Work out the finished part from the listing and answer in its coordinate system (mm). A direction names the side the tool comes from. Give positions to 0.01 mm unless a question says otherwise; leave off trailing zeros. Loops run counter-clockwise (first coordinate to the right, second up) from the corner with the lowest first, then second, coordinate; pieces in that order, holes last.
```python
from build123d import *

# Parameters (mm, degrees)
F0_W      = 82.55
F0_H      = 63.5
F1_DEPTH  = 15.748
F3_DEPTH  = 4.064
F4_W      = 19.05
F4_H      = 63.5
F5_DEPTH  = 4.826
F7_DEPTH  = 19.05
F8_R      = 6.35
F9_DEPTH  = 8.89
F14_DEPTH = 25.4
F16_DEPTH = 25.4
F18_W     = 23.9344900474
F18_H     = 17.6518000662
F19_DEPTH = 31.75


with BuildPart() as f1:
    # F0 (on Top) → F1 (new body)
    with BuildSketch(Plane.XY):
        Rectangle(F0_W, F0_H)
    extrude(amount=F1_DEPTH)

    # F2 (on face) → F3 (cut)
    with BuildSketch(Plane.XY.offset(15.748)):
        Polygon((-41.275, 1.4794587481), (-15.875, 31.75), (-41.275, 31.75), align=None)
    extrude(amount=-F3_DEPTH, mode=Mode.SUBTRACT)

    # F4 (on face) → F5 (join)
    with BuildSketch(Plane(origin=(0, 0, 0), x_dir=(1, 0, 0), z_dir=(0, 0, -1))):
        Rectangle(F4_W, F4_H)
    extrude(amount=F5_DEPTH)

    # F6 (on face) → F7 (join)
    with BuildSketch(Plane.XY.offset(15.748)):
        Polygon((41.275, -31.75), (41.275, 31.75), (34.925, 31.75), (-18.3578265798, -31.75), align=None)
    extrude(amount=F7_DEPTH)

    # F8 (on face) → F9 (cut)
    with BuildSketch(Plane.XY.offset(15.748)):
        with Locations((3.175, 12.7)):
            Circle(F8_R)
    extrude(amount=-F9_DEPTH, mode=Mode.SUBTRACT)

    # F13 (on face) → F14 (cut)
    with BuildSketch(Plane(origin=(0, -17.0362972024, 29.5082354343), x_dir=(1, 0, 0), z_dir=(0, 0.4999936063, -0.8660290951))):
        Polygon((-18.5759086162, 20.4719938338), (-20.111516118, 17.1120017767), (0, -10.4399453849), (43.6191521585, -10.4399453849), (43.6191521585, 20.4719938338), align=None)
    extrude(amount=-F14_DEPTH, mode=Mode.SUBTRACT)

    # F15 (on face) → F16 (cut)
    with BuildSketch(Plane(origin=(4.8610082234, -4.0788702074, 0), x_dir=(-0.6427876097, -0.7660444431, 0), z_dir=(-0.7660444431, 0.6427876097, 0))):
        Polygon((36.1220945353, 34.798), (14.8864189693, 34.798), (36.1220945353, 25.5741356141), align=None)
    extrude(amount=-F16_DEPTH, mode=Mode.SUBTRACT)

    # F18 (on offset) → F19 (cut)
    with BuildSketch(Plane(origin=(-41.275, 0, 0), x_dir=(0, -1, 0), z_dir=(-1, 0, 0))):
        with Locations((27.5025297888, 24.5739000331)):
            Rectangle(F18_W, F18_H)
    extrude(amount=-F19_DEPTH, mode=Mode.SUBTRACT)


solid = f1.part
```
Q1. Section B-B on z = 9 is taken. Give the vertices of the cut face in (x, y) (3 decimals), plus the area to 3 significant figures.
Q2. Section C-C on y = 24 is taken. Give the vertices of the cut face in (x, z) (3 decimals), plus the area to 3 significant figures.
Q3. Which of the six approach directions +Z, -Z, +X, -X, +Y, -Y give full straight-line access (tool end or side, diameter ignored) to faces 5 (the face through (-26, 0, 0)), 6 (the face through (-12, 0, 15.748)), 7 (the face through (25, 0, 0))?
Q4. Given pin 1 (1.4 mm diameter, centred on y = 9.5, z = -1.5, fed in from +X) (3 decimals); pin 2 (14.5 mm diameter, centred on x = 3.175, y = 12.7, fed in from +Z); pin 3 (6 mm diameter, centred on x = -13.5, y = 16.5, fed in from -Z), each flat-ended and moving along its own axis, determine where each tip first touches the part or whether it passes through.
Q5. Section A-A on x = 32.5 is taken. Give the vertices of the cut face in (y, z) (3 decimals), plus the area to 3 significant figures.
Q6. Determine the mould class of faces 1 (the face through (-9.525, -25, 20)), 2 (the face through (-1, -31.75, 8)), 3 (the face through (3, 13, 6.858)), 4 (the face through (10, 31.75, 10)) for opening direction Y: +Y half, -Y half, draft (parallel to the pull), parting line (faces both ways), or undercut.
Q7. Consider line 1 along Z through (x, y) = (-33, -25.5); line 2 along Z through (x, y) = (-1, 28.5); line 3 along X through (y, z) = (-13, -2) (3 decimals). Determine where each line is inside the solid, lowest interval first.
Q8. Section D-D on y = -4 is taken. Give the vertices of the cut face in (x, z) (3 decimals).
Check result:
1. outline: (-41.275, -31.75) - (41.275, -31.75) - (41.275, 31.75) - (-41.275, 31.75) - close; hole circle Ø12.7 at (3.175, 12.7)
1. area: 5,120 mm2
2. outline: (-41.275, 0) - (-9.525, 0) - (-9.525, -4.826) - (9.525, -4.826) - (9.525, 0) - (41.275, 0) - (41.275, 34.798) - (28.422, 34.798) - (28.422, 15.748) - (-22.378, 15.748) - (-22.378, 11.684) - (-41.275, 11.684) - close
2. area: 1,560 mm2
3. face 5: -Z, -X, +Y, -Y
3. face 6: +Z, -X, +Y
3. face 7: -Z, +X, +Y, -Y
4. pin 1: stops at x = 9.525
4. pin 2: stops at z = 15.75
4. pin 3: stops at z = 0
5. outline: (-31.75, 0) - (31.75, 0) - (31.75, 15.748) - (28.86, 15.748) - (28.86, 34.798) - (-8.035, 34.798) - (-7.995, 34.728) - (-31.75, 21.013) - close
5. area: 1,990 mm2
6. face 1: draft
6. face 2: -Y half
6. face 3: undercut
6. face 4: +Y half
7. line 1: z = 0 to 15.75
7. line 2: z = -4.83 to 15.75
7. line 3: x = -9.525 to 9.525
8. outline: (-41.275, 0) - (-9.525, 0) - (-9.525, -4.826) - (9.525, -4.826) - (9.525, 0) - (41.275, 0) - (41.275, 34.798) - (4.927, 34.798) - (4.927, 15.748) - (-41.275, 15.748) - close
